Answer from the drawing. Dimensions are ordinates in mm from the lowest x, y and z of the part. Round coordinates to 2 decimals unless told otherwise and drop trailing zeros. Write each loop counter-clockwise with the first axis right and the second up, starting at its lowest first coordinate (ties: lowest second). Pieces come first, ordered by that corner, then holes. Notation, with made-up numbers: (20, 14.25) - (45, 14.25) arc R29 cw to (45, 41.25) - close; hole circle Ø11 at (0.25, 59.5). An arc over 180 degrees is marked (long way). Answer as a JSON object with one key per item and string values.
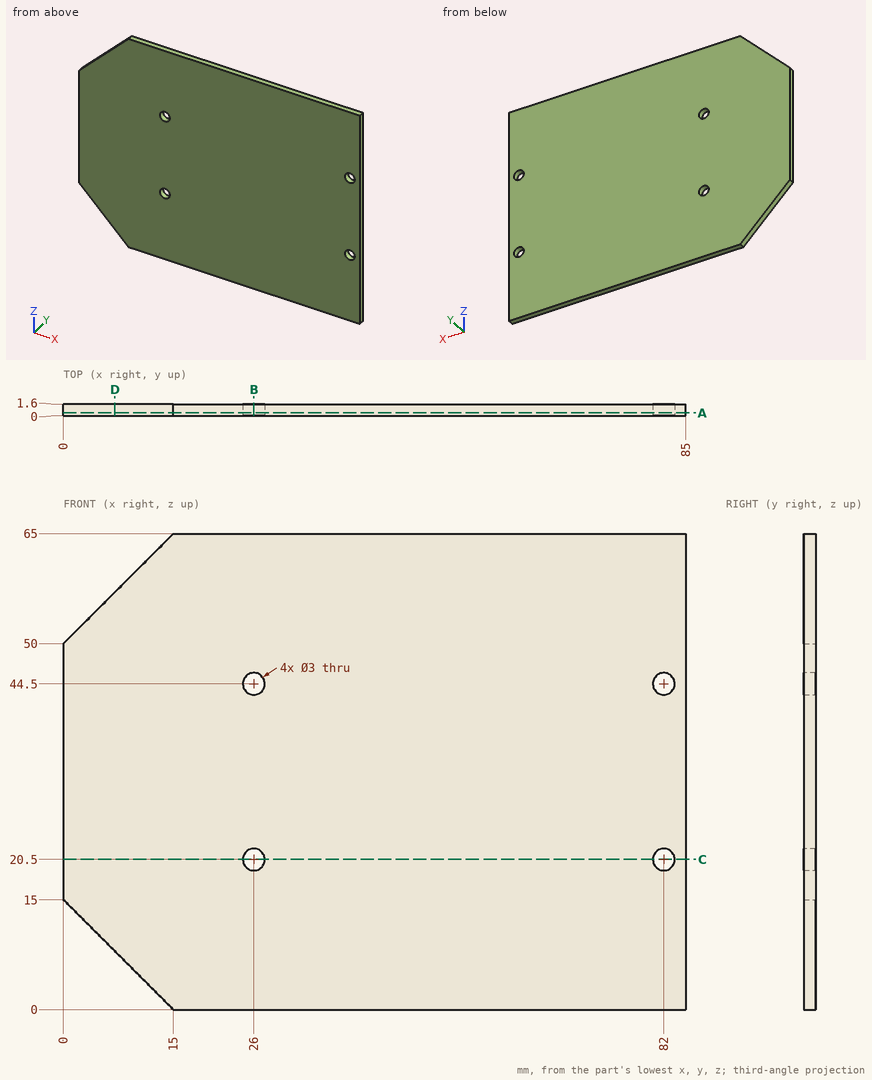
Item 1: A cutting plane is placed at C-C (z = 20.5). Write down the section's boundary in (x, y), and give its area (3 significant figures).
Results found:
{"outline": "(0, 0) - (24.5, 0) - (24.5, 1.6) - (0, 1.6) - close; (27.5, 0) - (80.5, 0) - (80.5, 1.6) - (27.5, 1.6) - close; (83.5, 0) - (85, 0) - (85, 1.6) - (83.5, 1.6) - close", "area": "126 mm²"}
Item 2: This flat-tipped pin is pushed along its axis until it touches: P1, Ø1.8, axis at x = 82, z = 20.5, coming from the +Y side. Where does it stop, or does it pass through?
Results found:
{"P1": "through"}
Item 3: A cutting plane is placed at D-D (x = 7). Write down the section's boundary in (y, z), and give its area (3 significant figures).
Results found:
{"outline": "(0, 8) - (1.6, 8) - (1.6, 57) - (0, 57) - close", "area": "78.4 mm²"}
Item 4: A cutting plane is placed at A-A (y = 0.4). Write down the section's boundary in (x, z), and give its area (3 significant figures).
Results found:
{"outline": "(0, 15) - (15, 0) - (85, 0) - (85, 65) - (15, 65) - (0, 50) - close; hole circle Ø3 at (26, 20.5); hole circle Ø3 at (26, 44.5); hole circle Ø3 at (82, 20.5); hole circle Ø3 at (82, 44.5)", "area": "5,270 mm²"}
Item 5: Consider line 1 along X through (y, z) = (0.85, 20.5); line 2 along Z through (x, y) = (82, 0.9); line 3 along X through (y, z) = (0.8, 44). Determine where each line is inside the solid, lowest interval first.
Results found:
{"line 1": "0 to 24.5, 27.5 to 80.5, 83.5 to 85", "line 2": "0 to 19, 22 to 43, 46 to 65", "line 3": "0 to 24.59, 27.41 to 80.59, 83.41 to 85"}
Item 6: A cutting plane is placed at B-B (x = 26). Write down the section's boundary in (y, z), and give its area (3 significant figures).
Results found:
{"outline": "(0, 0) - (1.6, 0) - (1.6, 19) - (0, 19) - close; (0, 22) - (1.6, 22) - (1.6, 43) - (0, 43) - close; (0, 46) - (1.6, 46) - (1.6, 65) - (0, 65) - close", "area": "94.4 mm²"}
